Autodesk Inventor part; units mm, degrees
ref_plane "Work Plane2" through (0, 0, 3) normal (0, 0, 1) x (1, 0, 0)
ref_plane "Work Plane3" through (0, 0, 3) normal (0, 0, 1) x (1, 0, 0)
ref_plane "YZ Plane" through (0, 0, 0) normal (1, 0, 0) x (0, 1, 0)
sketch "Sketch1" plane through (0, 0, 0) normal (0, 0, 1) x (1, 0, 0)
  line L0 (0, 0) -> (34, 0)
  line L1 (34, 0) -> (34, 19)
  line L2 (34, 19) -> (0, 19)
  line L3 (0, 19) -> (0, 0)
  dimension "d0" = 34
extrude "Extrusion1" add sketch "Sketch1" along normal blind 2
fillet "Fillet1" radius 2 4 edges at (34, 19, 1) (34, 0, 1) (0, 19, 1) (0, 0, 1)
sketch "Sketch3" plane through (0, 2, 0) normal (-1, 0, 0) x (0, 0, 1)
  line L0 (2, 0) -> (0, 0) construction
  line L1 (2, 15) -> (2, 0) construction
  line L2 (0, 0) -> (2, 15) construction
  line L3 (0, 15) -> (2, 0) construction
  circle A0 centre (1, 7.5) radius 2
  point P0 (0, -2)
  dimension "d4" = 4
extrude "Extrusion2" add sketch "Sketch3" along normal blind 2 and the other way blind 10
sketch "Sketch4" plane through (-2, 9.5, 1) normal (-1, 0, 0) x (0, 0, 1)
  point P0 (-1, -9.5)
  point P1 (0, 0)
hole "Hole1" at (-2, 9.5, 1) direction (1, 0, 0) diameter 2.85 depth 10.4 tip angle 118
ref_plane "Work Plane2" through (0, 0, 3) normal (0, 0, 1) x (1, 0, 0)
ref_plane "Work Plane1" through (0, 0, 1) normal (0, 0, 1) x (1, 0, 0)
sketch "Sketch6" plane through (0, 0, 3) normal (0, 0, 1) x (1, 0, 0)
  line L0 (-2, 11.5) -> (-2, 7.5) construction
  line L1 (0, 7.5) -> (0, 7.7679) construction
  line L2 (-2, 11.5) -> (0, 7.5) construction
  line L3 (0, 7.5) -> (-2, 7.5) construction
  line L4 (-2, 7.5) -> (0, 11.5) construction
  line L5 (0, 11.5) -> (-2, 11.5) construction
  point P0 (0, 0)
  point P1 (-1, 9.5)
hole "Hole2" at (-1, 9.5, 3) direction (0, 0, -1) diameter 1 end through all
ref_plane "Work Plane3" through (0, 0, 3) normal (0, 0, 1) x (1, 0, 0)
properties part number "UntererRührerBlatt"
Geometry: final body of the model. Coordinates: model frame, mm. A direction names the side the tool comes from. Round coordinates to 2 decimals unless told otherwise and drop trailing zeros. Loops run counter-clockwise (first coordinate to the right, second up) from the corner with the lowest first, then second, coordinate; pieces in that order, holes last. Notation, with made-up numbers: (57.5, -24.5) - (116.5, -24.5) arc R29 ccw to (116.5, 8.5) - close; hole circle Ø2 at (-7.5, 68.5). An arc over 180 degrees is marked (long way). Write each question's results on one line, items separated by ' | '. Start each with the question number.
1) Cut plane A-A on x = 7. Return loops of the section in (y, z) (3 decimals), then the cut area to 3 significant figures.
2) Line query: probe 1 along Z at (x, y) = (1, 9.5) (3 decimals); probe 2 along X at (y, z) = (9.5, 2.5); probe 3 along Y at (x, z) = (6, 1) (3 decimals). Output: solid intervals per line, ascending. Write a range as [from, to].
3) Access query for faces 1 (the face through (10, 9.5, 2.4)), 2 (the face through (-2, 8, 2)). Directions: +Z, -Z, +X, -X, +Y, -Y. A direction counts if a zero-diameter tool reaches every point of the face in a straight line with its end or side. Return the directions, or none.
4) Mould query, pull axis Z, two halves, no side actions, for faces 3 (the face through (3.27, 9.07, 2.36)), 4 (the face through (17, 10, 0)), 5 (the face through (10, 9.5, -0.4)). Classes: released by +Z, released by -Z, zero draft, split by the parting line, or undercut.
5) First-contact query: P1, Ø10, axis at x = 30.5, y = 10.5, coming from the +Z side; P2, Ø0.5, axis at y = 10, z = -0.5, coming from the +X side; P3, Ø4, axis at x = 19, y = 12, coming from the -Z side; P4, Ø3, axis at x = 10, y = 10.5, coming from the +Z side. Flat tips, straight axial feed; report the tip coordinate or a pass-through.
6) Cut plane D-D on x = 26. Return loops of the section in (y, z), then the cut area to 3 significant figures.
7) Cut plane B-B on y = 4.5. Return loops of the section in (x, z), then the cut area to 3 significant figures.
Verdict:
1) outline: (0, 0) - (7.768, 0) arc R2 ccw to (11.232, 0) - (19, 0) - (19, 2) - (11.232, 2) arc R2 ccw to (7.768, 2) - (0, 2) - close; hole circle Ø2.85 at (9.5, 1) | area: 36.5 mm2
2) probe 1: z = [-1, -0.425], [2.425, 3] | probe 2: x = [-2, -1.5], [-0.5, 10] | probe 3: y = [0, 8.075], [10.925, 19]
3) face 1: +Z, +X, +Y, -Y | face 2: +Z, -Z, -X, +Y, -Y
4) face 3: undercut | face 4: released by -Z | face 5: zero draft
5) P1: stops at z = 2 | P2: stops at x = 10 | P3: stops at z = 0 | P4: stops at z = 3
6) outline: (0, 0) - (19, 0) - (19, 2) - (0, 2) - close | area: 38.0 mm2
7) outline: (0, 0) - (34, 0) - (34, 2) - (0, 2) - close | area: 68.0 mm2
